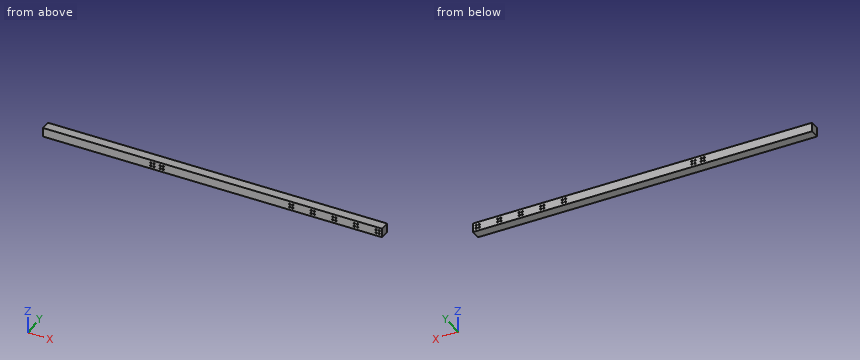
```python
from build123d import *

# Parameters (mm, degrees)
F0_W     = 1100
F0_H     = 30
F1_DEPTH = 15
F3_D     = 5


with BuildPart() as f1:
    # F0 (on Front) → F1 (new body, symmetric)
    with BuildSketch(Plane.XZ):
        Rectangle(F0_W, F0_H)
    extrude(amount=F1_DEPTH, both=True)

    # F3 (through all)
    with Locations(Plane.XZ.offset(15)):
        with Locations((-170, 5), (-170, -5), (-160, -5), (-160, 5), (530, 5), (530, -5), (540, 5), (540, -5), (470, 5), (460, 5), (460, -5), (470, -5), (250, 5), (250, -5), (260, -5), (260, 5), (320, 5), (320, -5), (330, -5), (330, 5), (390, 5), (390, -5), (400, -5), (400, 5), (-190, 5), (-200, 5), (-200, -5), (-190, -5)):
            Hole(F3_D / 2)


solid = f1.part
```
Source: CAD feature listing. Evaluate the final solid. Frame: model axes, mm. Round coordinates to 2 decimals unless told otherwise and drop trailing zeros.
1. Contact query for a flat-ended pin moving along its axis: pin 1 (4 mm diameter, centred on x = 390, z = 5, fed in from -Y). Output: stop coordinate, or through.
2. Section query A-A on y = 10.5. Give the number of separate pieces and of enclosed holes in the cut face, and give its area (3 significant figures).
3. Ray query, L1, parallel to Z at x = 329, y = -6.25; L2, parallel to Z at x = 530, y = 3.25. Return the intervals inside material, ascending.
Answers below:
1. pin 1: passes through
2. separate pieces: 1
2. enclosed holes: 28
2. area: 32,500 mm2
3. L1: z = -15 to -7.29, -2.71 to 2.71, 7.29 to 15
3. L2: z = -15 to -7.5, -2.5 to 2.5, 7.5 to 15
